from build123d import *

# Parameters (mm, degrees)
F0_R     = 25
F1_DEPTH = 35


with BuildPart() as f1:
    # F0 (on Top) → F1 (new body)
    with BuildSketch(Plane.XY):
        Circle(F0_R)
    extrude(amount=F1_DEPTH)

    # F2 (on Front) → F3 (revolve, cut)
    with BuildSketch(Plane.XZ):
        with BuildLine():
            Line((-12.442632, 24.75), (-25, 32))
            Line((-25, 32), (-25, 3))
            Line((-25, 3), (-12.442632, 10.25))
            ThreePointArc((-12.442632, 10.25), (-10.5, 17.5), (-12.442632, 24.75))
        make_face()
    revolve(axis=Axis((0, 0, 17.5), (0, 0, 1)), mode=Mode.SUBTRACT)


solid = f1.part
Model file for the job. Use its own axes, mm. A direction names the side the tool comes from. Give positions to 0.01 mm unless a question says otherwise; leave off trailing zeros. Loops run counter-clockwise (first coordinate to the right, second up) from the corner with the lowest first, then second, coordinate; pieces in that order, holes last. Notation, with made-up numbers: (67.25, 10.25) -> (112.25, 10.25) arc R15 ccw to (112.25, 32.25) -> close; hole circle Ø6 at (61.25, -35). An arc over 180 degrees is marked (long way). Use a Markdown table: item, result. Add a question column.
(1) Slice it at D-D on z = 18. List the corners of the cut face in (x, y), and give its area (3 significant figures).
(2) Slice it at C-C on z = 6. List the corners of the cut face in (x, y), and give its area (3 significant figures).
(3) Drop flat-ended pins along their axis: pin 1 Ø5 at (y, z) = (10.5, 15) entering from -X; pin 2 Ø12 at (y, z) = (2.5, 24) entering from +X; pin 3 Ø12 at (x, z) = (5, 14.5) entering from +Y. Give the stop position or say it passes through.
(4) Slice it at A-A on x = 0. List the corners of the cut face in (y, z), and give its area (3 significant figures).
(5) Tool access for faces 1 (the flat face through (0, 0, 0)), 2 (the conical face through (2.9, 12.9, 25.2)): list every direction of +Z, -Z, +X, -X, +Y, -Y with a clear straight run to the whole face (end or side of a thin tool).
(6) Wall check: line 1 along Z through (x, y) = (-14, -8.5); line 2 along Z through (x, y) = (5.5, 13); line 3 along Y through (x, z) = (-10.5, 8). Give the ranges that are in metal, low to high.
Filled sheet:
| question | item | result |
|---|---|---|
| 1 | outline | circle Ø21.02 at (0, 0) |
| 1 | area | 347 mm2 |
| 2 | outline | circle Ø39.61 at (0, 0) |
| 2 | area | 1,230 mm2 |
| 3 | pin 1 | x = -7.23 |
| 3 | pin 2 | x = 21.41 |
| 3 | pin 3 | y = 14.8 |
| 4 | outline | (-25, 0) -> (25, 0) -> (25, 3) -> (12.44, 10.25) arc R14.5 cw to (12.44, 24.75) -> (25, 32) -> (25, 35) -> (-25, 35) -> (-25, 32) -> (-12.44, 24.75) arc R14.5 cw to (-12.44, 10.25) -> (-25, 3) -> close |
| 4 | area | 1,170 mm2 |
| 5 | face 1 | -Z, +X, -X, +Y, -Y |
| 5 | face 2 | none |
| 6 | line 1 | 0 to 7.98, 27.02 to 35 |
| 6 | line 2 | 0 to 9.28, 25.72 to 35 |
| 6 | line 3 | -12.52 to 12.52 |
